Job drawing, mm, ordinate dimensions from the low corner. One solid piece. Give positions to 0.01 mm unless a question says otherwise; leave off trailing zeros. Write each loop counter-clockwise with the first axis right and the second up, starting at its lowest first coordinate (ties: lowest second). Pieces come first, ordered by that corner, then holes. Notation, with made-up numbers: (1, 18) - (5, 18) arc R31 ccw to (5, 43) - close; hole circle Ø7 at (47, 68). An arc over 180 degrees is marked (long way). Answer as a JSON object with one key per item and string values.
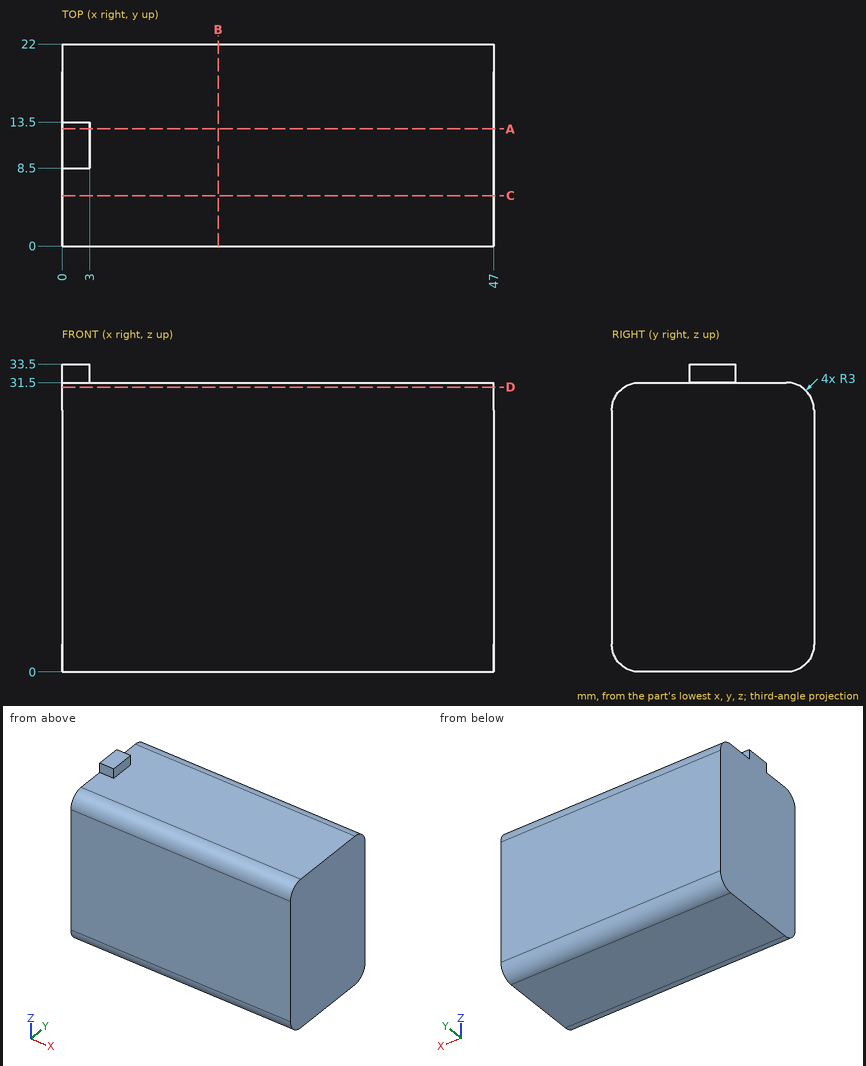
Item 1: Cut at D-D (z = 31). Give the cut face in (x, y), and give its area (3 significant figures).
Entries:
{"outline": "(0, 1.34) - (47, 1.34) - (47, 20.66) - (0, 20.66) - close", "area": "908 mm2"}
Item 2: Probe line 1 (Z direction, x = 38, y = 9.25); line 2 (Z direction, x = 17.5, y = 20.25); line 3 (Y direction, x = 13, z = 30.5). List the from-to ranges inside material, lowest first. Write a range as from..to.
Entries:
{"line 1": "0..31.5", "line 2": "0.27..31.23", "line 3": "0.76..21.24"}
Item 3: Cut at A-A (y = 12.75). Give the cut face in (x, z).
Entries:
{"outline": "(0, 0) - (47, 0) - (47, 31.5) - (3, 31.5) - (3, 33.5) - (0, 33.5) - close"}
Item 4: Cut at C-C (y = 5.5). Give the cut face in (x, z), and give its area (3 significant figures).
Entries:
{"outline": "(0, 0) - (47, 0) - (47, 31.5) - (0, 31.5) - close", "area": "1,480 mm2"}
Item 5: Flat gauge pins, fed straight in: P1, Ø6, axis at y = 6, z = 17, coming from the -X side; P2, Ø8, axis at x = 33.5, y = 14.5, coming from the +Z side; P3, Ø2, axis at y = 11, z = 33, coming from the +X side; P4, Ø0.6, axis at x = 2, z = 32.5, coming from the +Y side. Where does each tip first touch, or does it go through?
Entries:
{"P1": "x = 0", "P2": "z = 31.5", "P3": "x = 3", "P4": "y = 13.5"}
Item 6: Cut at B-B (x = 17). Give the cut face in (y, z).
Entries:
{"outline": "(0, 3) arc R3 ccw to (3, 0) - (19, 0) arc R3 ccw to (22, 3) - (22, 28.5) arc R3 ccw to (19, 31.5) - (3, 31.5) arc R3 ccw to (0, 28.5) - close"}
